Check sheet for the modelled part. Datum: model origin and axes. Units: mm. Face numbers are marked on the shaded views. A direction names the side the tool comes from. Round coordinates to 2 decimals unless told otherwise and drop trailing zeros. Loops run counter-clockwise (first coordinate to the right, second up) from the corner with the lowest first, then second, coordinate; pieces in that order, holes last. Notation, with made-up numbers: (8, 11) - (49, 11) arc R29 ccw to (49, 44) - close; hole circle Ø7 at (20.5, 40.25). An arc over 180 degrees is marked (long way). Answer in a Markdown table with one row per item. Add a question column.
(1) Mould release check, pull along Z, two halves, no side actions. Record for the marked faces 3, 4, 5 and 6: +Z half, -Z half, draft (parallel to the pull), parting line (faces both ways), or undercut.
(2) Gauge pin test, flat ends, axial feed: pin 1 (3.5 mm diameter, centred on y = 5, z = -66, fed in from +X); pin 2 (22.5 mm diameter, centred on x = -12, y = 29.5, fed in from -Z); pin 3 (4 mm diameter, centred on x = 74.5, y = 29.5, fed in from -Z); pin 4 (2.5 mm diameter, centred on x = -74, y = 31, fed in from -Z). Record the tip position at first contact, or that the pin passes through.
(3) Cross-section at A-A on z = 35. Enter the section's corners in (x, y).
(4) Thickness scan on line 1 along X through (y, z) = (38, -52.5); line 2 along X through (y, z) = (38, -56.5); line 3 along X through (y, z) = (9, -50). Record the ranges inside material, lowest first.
(5) Access from +Z, -Z, +X, -X, +Y, -Y to the whole of each face (thin tool, end or side, straight path). Record for the marked faces 1 and 2.
(6) Cross-section at D-D on z = -1. Enter the section's corners in (x, y).
(7) Cross-section at B-B on x = -49. Enter the section's corners in (y, z).
(8) Cross-section at C-C on y = 5. Count the separate pieces of the cut face and the enclosed holes in it, then the cut area to 3 significant figures.
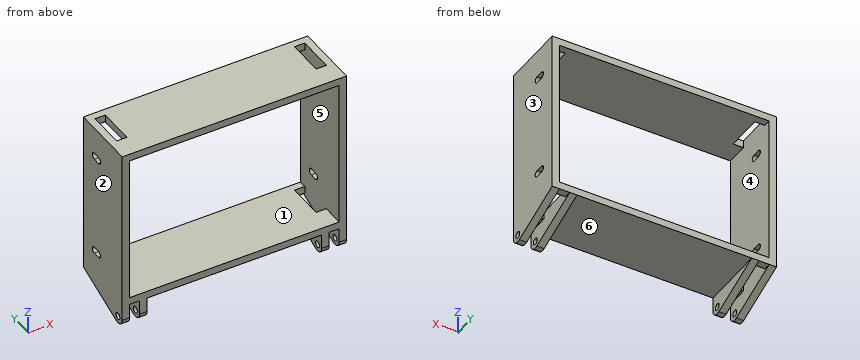
from build123d import *

# Parameters (mm, degrees)
SKETCH1_W               = 154
SKETCH1_H               = 112
SKETCH1_W_2             = 144
SKETCH1_H_2             = 102
BOSS_EXTRUDE1_DEPTH     = 45
CUT_EXTRUDE1_DEPTH      = 180.5
SKETCH3_W               = 7
SKETCH3_H               = 25
CUT_EXTRUDE3_DEPTH      = 134
SKETCH4_R               = 2.25
BOSS_EXTRUDE2_DEPTH     = 5
LPATTERN1_COUNT         = 2
LPATTERN1_PITCH         = 12
MIRROR1_COPY_1_SKETCH_R = 2.25
MIRROR1_COPY_1_DEPTH    = 5


with BuildPart() as part:
    # Sketch1 → Boss-Extrude1 (new body)
    with BuildSketch(Plane(origin=(0, 0, 0), x_dir=(1, 0, 0), z_dir=(0, 1, 0))):
        Rectangle(SKETCH1_W, SKETCH1_H)
        Rectangle(SKETCH1_W_2, SKETCH1_H_2, mode=Mode.SUBTRACT)
    extrude(amount=BOSS_EXTRUDE1_DEPTH)

    # Sketch2 → Cut-Extrude1 (cut)
    with BuildSketch(Plane.ZY.offset(77)):
        with BuildLine():
            Line((-32.75, 32.5), (-32.75, 27.5))
            ThreePointArc((-32.75, 27.5), (-35, 25.25), (-37.25, 27.5))
            Line((-37.25, 27.5), (-37.25, 32.5))
            ThreePointArc((-37.25, 32.5), (-35, 34.75), (-32.75, 32.5))
        make_face()
        with BuildLine():
            Line((37.25, 32.5), (37.25, 27.5))
            ThreePointArc((37.25, 27.5), (35, 25.25), (32.75, 27.5))
            Line((32.75, 27.5), (32.75, 32.5))
            ThreePointArc((32.75, 32.5), (35, 34.75), (37.25, 32.5))
        make_face()
    extrude(amount=-CUT_EXTRUDE1_DEPTH, mode=Mode.SUBTRACT)

    # Sketch3 → Cut-Extrude3 (cut)
    with BuildSketch(Plane(origin=(0, 0, -56), x_dir=(-1, 0, 0), z_dir=(0, 0, -1))):
        with Locations((-68.5, 27.5)):
            Rectangle(SKETCH3_W, SKETCH3_H)
        with Locations((68.5, 27.5)):
            Rectangle(SKETCH3_W, SKETCH3_H)
    extrude(amount=-CUT_EXTRUDE3_DEPTH, mode=Mode.SUBTRACT)

    # Sketch4 → Boss-Extrude2 (add)
    with BuildSketch(Plane.ZY.offset(77)):
        with BuildLine():
            Line((-66, 0), (-56, 0))
            Line((-56, 0), (-56, 45))
            Line((-56, 45), (-70.667854572, 6.791963643))
            ThreePointArc((-70.667854572, 6.791963643), (-70.120668527, 2.168023501), (-66, 0))
        make_face()
        with Locations((-66, 5)):
            Circle(SKETCH4_R, mode=Mode.SUBTRACT)
    boss_extrude2 = extrude(amount=-BOSS_EXTRUDE2_DEPTH)

    # LPattern1: Boss-Extrude2 ×2
    with Locations(*[(i * LPATTERN1_PITCH, 0, 0) for i in range(1, LPATTERN1_COUNT)]):
        add(boss_extrude2)

    # Mirror1: Boss-Extrude2 across plane
    add(boss_extrude2.mirror(Plane(origin=(0, 0, 0), x_dir=(0, 0, 1), z_dir=(1, 0, 0))))

    # Mirror1 copy 1 sketch → Mirror1 copy 1 (add)
    with BuildSketch(Plane(origin=(65, 0, 0), x_dir=(0, 0, 1), z_dir=(1, 0, 0))):
        with BuildLine():
            Line((-66, 0), (-56, 0))
            Line((-56, 0), (-56, -45))
            Line((-56, -45), (-70.667854572, -6.791963643))
            ThreePointArc((-70.667854572, -6.791963643), (-70.120668527, -2.168023501), (-66, 0))
        make_face()
        with Locations((-66, -5)):
            Circle(MIRROR1_COPY_1_SKETCH_R, mode=Mode.SUBTRACT)
    extrude(amount=-MIRROR1_COPY_1_DEPTH)


solid = part.part
Answers:
| question | item | result |
|---|---|---|
| 1 | face 3 | draft |
| 1 | face 4 | undercut |
| 1 | face 5 | undercut |
| 1 | face 6 | -Z half |
| 2 | pin 1 | passes through |
| 2 | pin 2 | stops at z = -56 |
| 2 | pin 3 | stops at z = -62.72 |
| 2 | pin 4 | stops at z = -61.85 |
| 3 | outline | (-77, 0) - (-72, 0) - (-72, 25.25) - (-77, 25.25) - close; (-77, 34.75) - (-72, 34.75) - (-72, 45) - (-77, 45) - close; (72, 0) - (77, 0) - (77, 25.25) - (72, 25.25) - close; (72, 34.75) - (77, 34.75) - (77, 45) - (72, 45) - close |
| 4 | line 1 | x = -77 to -72, -65 to 65, 72 to 77 |
| 4 | line 2 | x = -77 to -72, -65 to -60, 60 to 65, 72 to 77 |
| 4 | line 3 | x = -77 to -72, 72 to 77 |
| 5 | face 1 | +Y, -Y |
| 5 | face 2 | +Z, -Z, -X, +Y, -Y |
| 6 | outline | (-77, 0) - (-72, 0) - (-72, 45) - (-77, 45) - close; (72, 0) - (77, 0) - (77, 45) - (72, 45) - close |
| 7 | outline | (0, -56) - (45, -56) - (45, -51) - (0, -51) - close; (0, 51) - (45, 51) - (45, 56) - (0, 56) - close |
| 8 | separate pieces | 5 |
| 8 | enclosed holes | 1 |
| 8 | area | 2,770 mm^2 |
